The model under review builds one solid part; all positions refer to its coordinate system, in mm. Give positions to 0.01 mm unless a question says otherwise; leave off trailing zeros. Loops run counter-clockwise (first coordinate to the right, second up) from the corner with the lowest first, then second, coordinate; pieces in that order, holes last. Notation, with made-up numbers: M -23,47 L -4,47 A24 cw -4,61 Z; hole C 1,14 d10. An arc over 180 degrees is marked long. Return JSON: item names as keys, results as strings. Group by question number.
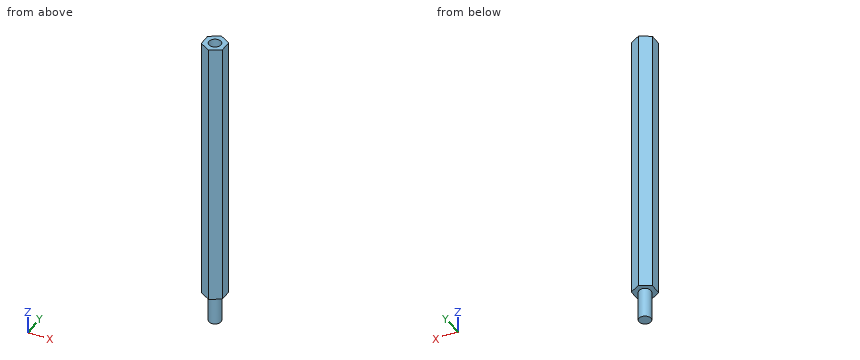
Autodesk Inventor part; units mm, degrees
ref_plane "YZ Plane" through (0, 0, 0) normal (1, 0, 0) x (0, 1, 0)
ref_plane "XZ Plane" through (0, 0, 0) normal (0, 1, 0) x (-1, 0, 0)
ref_plane "XY Plane" through (0, 0, 0) normal (0, 0, 1) x (1, 0, 0)
sketch "スケッチ1" plane through (0, 0, 0) normal (0, 0, 1) x (1, 0, 0)
  circle A0 centre (0, 0) radius 3.5 construction
  line L0 (3.5, -2.0207) -> (0, -4.0415)
  line L1 (0, -4.0415) -> (-3.5, -2.0207)
  line L2 (-3.5, -2.0207) -> (-3.5, 2.0207)
  line L3 (-3.5, 2.0207) -> (0, 4.0415)
  line L4 (0, 4.0415) -> (3.5, 2.0207)
  line L5 (3.5, 2.0207) -> (3.5, -2.0207)
  point P0 (3.5, 0)
  dimension "d0" = 7
extrude "押し出し1" add sketch "スケッチ1" along normal blind 90
sketch "スケッチ2" plane through (0, 0, 90) normal (0, 0, 1) x (1, 0, 0)
  point P0 (0, 0)
  point P1 (0, 0)
hole "穴1" at (0, 0, 90) direction (0, 0, -1) diameter 4 depth 12 tip angle 118
sketch "スケッチ3" plane through (0, 0, 0) normal (0, 0, -1) x (-1, 0, 0)
  circle A0 centre (0, 0) radius 2
  dimension "d10" = 4
extrude "押し出し2" add sketch "スケッチ3" along normal blind 10
properties part number "六角スペーサー"
(1) Add section B-B (z = -2.5). Write out the cut boundary in (x, y).
(2) Add section A-A (z = 70). Write out the cut boundary in (x, y), and give its area (3 significant figures).
(3) For probe 1 along Y at (x, z) = (0, 80.75); probe 2 along X at (y, z) = (0, 81.75); probe 3 along Z at (x, y) = (-1.25, -2), list the stretches that pass through material, from the lowest coordinate up.
(4) For pin 1 (1 mm diameter, centred on x = 1.5, z = 16.5, fed in from +Y); pin 2 (3.5 mm diameter, centred on x = 0, y = 0, fed in from +Z), all flat-tipped, find the tip position at first contact; note any pin that passes through.
Verdict:
{
 "1": {"outline": "C 0,0 d4"},
 "2": {"outline": "M -3.5,-2.02 L 0,-4.04 L 3.5,-2.02 L 3.5,2.02 L 0,4.04 L -3.5,2.02 Z", "area": "42.4 mm²"},
 "3": {"probe 1": "y = -4.04 to -2, 2 to 4.04", "probe 2": "x = -3.5 to -2, 2 to 3.5", "probe 3": "z = 0 to 90"},
 "4": {"pin 1": "stops at y = 3.46", "pin 2": "stops at z = 77.85"}
}
